from build123d import *

# Parameters (mm, degrees)
BOSS_EXTRUDE1_DEPTH = 3.175
CUT_EXTRUDE1_DEPTH  = 46.236786745


with BuildPart() as part:
    # Sketch1 → Boss-Extrude1 (new body)
    with BuildSketch(Plane.XY):
        Polygon((-34.925, 28.575), (-34.925, -3.175), (-15.875, -3.175), (-15.875, 0), (15.875, 0), (15.875, -3.175), (34.925, -3.175), (34.925, 28.575), (27.432, 28.575), (27.432, 22.225), (-27.432, 22.225), (-27.432, 28.575), align=None)
    extrude(amount=BOSS_EXTRUDE1_DEPTH)

    # Sketch2 → Cut-Extrude1 (cut, through all)
    with BuildSketch(Plane.XY.offset(3.175)):
        with BuildLine():
            Line((-21.082, 22.225), (21.082, 22.225))
            ThreePointArc((21.082, 22.225), (0, 4.080259171), (-21.082, 22.225))
        make_face()
        Polygon((-28.575, 17.330749155), (-28.575, 2.090749155), (-15.875, 2.090749155), align=None)
        Polygon((28.575, 2.090749155), (15.875, 2.090749155), (28.575, 17.330749155), align=None)
    extrude(amount=-CUT_EXTRUDE1_DEPTH, mode=Mode.SUBTRACT)


solid = part.part
The listing builds one solid part. Answer for the finished solid, in the listing's coordinates (mm). A direction names the side the tool comes from. Round coordinates to 2 decimals unless told otherwise and drop trailing zeros. Loops run counter-clockwise (first coordinate to the right, second up) from the corner with the lowest first, then second, coordinate; pieces in that order, holes last. Notation, with made-up numbers: M 3.5,62.5 L 58.5,62.5 A21 cw 58.5,67.5 Z; hole C 85.5,-22.75 d8. An arc over 180 degrees is marked long. Write each question's results on one line, items separated by ' | '. Start each with the question number.
1) Each of these flat-tipped pins is pushed along its axis until it touches: pin 1 (1 mm diameter, centred on x = -13.5, z = 1.5, fed in from -Y); pin 2 (1 mm diameter, centred on x = -12, z = 2.5, fed in from +Y); pin 3 (1 mm diameter, centred on x = 25.5, z = 2.5, fed in from +Y) (3 decimals); pin 4 (8 mm diameter, centred on x = -4, y = 10.5, fed in from -Z). Where does it stop, or does it pass through?
2) Straight lines are drawn through the part: probe 1 along X at (y, z) = (6, 2.55) (3 decimals); probe 2 along X at (y, z) = (12.5, 3.05) (3 decimals); probe 3 along X at (y, z) = (4, 2.2) (3 decimals). For each, find the intervals that lie inside material, in ascending order.
3) Which of the six approach directions +Z, -Z, +X, -X, +Y, -Y give full straight-line access (tool end or side, diameter ignored) to faces 5 (the flat face through (-15.875, -2, 2)), 6 (the flat face through (-24, 22.225, 2)), 7 (the flat face through (22, 2.091, 2)), 8 (the flat face through (25, -3.175, 2))?
4) Determine the mould class of faces 1 (the cylindrical face through (0.424, 4.084, 1.61)), 2 (the flat face through (34.925, 12, 2)), 3 (the flat face through (-26, -3.175, 2)), 4 (the flat face through (-34.925, 13, 2)) for opening direction X: pulls with the +X half, pulls with the -X half, needs draft (parallel to the pull), parting line crosses it, or undercut.
5) Find section C-C on x = -24. Write down the section's boundary in (y, z) (3 decimals), plus the area to 3 significant figures.
6) Find section D-D on y = 5. Write down the section's boundary in (x, z) (3 decimals), plus the area to 3 significant figures.
7) Find section A-A on z = 1.2. Write down the section's boundary in (x, y) (3 decimals).
8) Find section B-B on y = 19.5. Write down the section's boundary in (x, z) (3 decimals).
Final values:
1) pin 1: y = 0 | pin 2: y = 8.13 | pin 3: y = 22.225 | pin 4: through
2) probe 1: -34.925 to -28.575, -19.133 to -8.841, 8.841 to 19.133, 28.575 to 34.925 | probe 2: -34.925 to -28.575, -24.549 to -16.974, 16.974 to 24.549, 28.575 to 34.925 | probe 3: -34.925 to -28.575, -17.466 to 17.466, 28.575 to 34.925
3) face 5: +Z, -Z, -Y | face 6: +Z, -Z, +Y | face 7: +Z, -Z | face 8: +Z, -Z, +X, -X, -Y
4) face 1: undercut | face 2: pulls with the +X half | face 3: needs draft | face 4: pulls with the -X half
5) outline: M -3.175,0 L 2.091,0 L 2.091,3.175 L -3.175,3.175 Z; M 11.841,0 L 22.225,0 L 22.225,3.175 L 11.841,3.175 Z | area: 49.7 mm²
6) outline: M -34.925,0 L -28.575,0 L -28.575,3.175 L -34.925,3.175 Z; M -18.299,0 L -6.194,0 L -6.194,3.175 L -18.299,3.175 Z; M 6.194,0 L 18.299,0 L 18.299,3.175 L 6.194,3.175 Z; M 28.575,0 L 34.925,0 L 34.925,3.175 L 28.575,3.175 Z | area: 117 mm²
7) outline: M -34.925,-3.175 L -15.875,-3.175 L -15.875,0 L 15.875,0 L 15.875,-3.175 L 34.925,-3.175 L 34.925,28.575 L 27.432,28.575 L 27.432,22.225 L 21.082,22.225 A21.32 cw -21.082,22.225 L -27.432,22.225 L -27.432,28.575 L -34.925,28.575 Z; hole M -28.575,2.091 L -15.875,2.091 L -28.575,17.331 Z; hole M 15.875,2.091 L 28.575,2.091 L 28.575,17.331 Z
8) outline: M -34.925,0 L -20.487,0 L -20.487,3.175 L -34.925,3.175 Z; M 20.487,0 L 34.925,0 L 34.925,3.175 L 20.487,3.175 Z
